Here's how the part is built. I have some questions about the finished solid (model axes, mm). A direction names the side the tool comes from. Coordinates: 2 decimals unless noted, no trailing zeros. Write each loop counter-clockwise with the first axis right and the second up, starting at its lowest first coordinate (ties: lowest second). Pieces come first, ordered by that corner, then holes.
Item 1: I want a section at B-B (x = 0). Please give me the cut outline in (y, z), and give its area (3 significant figures).
Item 2: I want a section at C-C (z = 53). Please give me the cut outline in (x, y) (1 decimal).
Item 3: I'm going to push flat-ended pins straight in: P1, Ø1.5, axis at x = -3.5, z = 65, coming from the +Y side; P2, Ø8, axis at x = -5, z = 20.5, coming from the -Y side; P3, Ø1.5, axis at x = -4.5, z = 24, coming from the +Y side; P4, Ø6, axis at x = 1, y = -1, coming from the -Z side. Where does each tip first touch, or does it pass through?
Item 4: Please list where these lines run through material, in increasing order: line 1 (Z direction, x = -4.5, y = -9); line 2 (Y direction, x = -3.5, z = 63); line 3 (Y direction, x = -6.5, z = 17.5).
Item 5: For faces 1 (the face through (1, -11.992, 79)), 2 (the face through (-1.72, 7.75, 37.57)), which set-ups out of +Z, -Z, +X, -X, +Y, -Y let a thin tool reach every point of the face, with its end or its side?
Item 6: I want a section at A-A (y = 0). Please give me the cut outline in (x, z), and give its area (3 significant figures).
Autodesk Inventor part; units mm, degrees
ref_plane "YZ Plane" through (0, 0, 0) normal (1, 0, 0) x (0, 1, 0)
ref_plane "XZ Plane" through (0, 0, 0) normal (0, 1, 0) x (-1, 0, 0)
ref_plane "XY Plane" through (0, 0, 0) normal (0, 0, 1) x (1, 0, 0)
sketch "Sketch1" plane through (0, 0, 0) normal (0, 0, 1) x (1, 0, 0)
  circle A0 centre (0, 0) radius 7.9375
  dimension "d0" = 15.875
extrude "Extrusion1" add sketch "Sketch1" along normal blind 76.2
sketch "Sketch2" plane through (0, 0, 76.2) normal (0, 0, 1) x (1, 0, 0)
  line L0 (-12.2432, 12.9979) -> (13.2495, 12.9979)
  line L1 (13.2495, 12.9979) -> (13.2495, -11.9916)
  line L2 (13.2495, -11.9916) -> (-12.2432, -11.9916)
  line L3 (-12.2432, -11.9916) -> (-12.2432, 12.9979)
  point P0 (0, 0)
extrude "Extrusion2" add sketch "Sketch2" along normal blind 6.5673
properties part number "KBOLT"
Answer:
1. outline: (-11.99, 76.2) - (-7.94, 76.2) - (-7.94, 0) - (7.94, 0) - (7.94, 76.2) - (13, 76.2) - (13, 82.77) - (-11.99, 82.77) - close
1. area: 1,370 mm2
2. outline: circle Ø15.9 at (0, 0)
3. P1: stops at y = 7.45
3. P2: stops at y = -7.87
3. P3: stops at y = 7
3. P4: stops at z = 0
4. line 1: z = 76.2 to 82.77
4. line 2: y = -7.12 to 7.12
4. line 3: y = -4.56 to 4.56
5. face 1: +Z, -Z, +X, -X, -Y
5. face 2: -Z
6. outline: (-12.24, 76.2) - (-7.94, 76.2) - (-7.94, 0) - (7.94, 0) - (7.94, 76.2) - (13.25, 76.2) - (13.25, 82.77) - (-12.24, 82.77) - close
6. area: 1,380 mm2
